The model under review builds one solid part; all positions refer to its coordinate system, in mm. A direction names the side the tool comes from. Coordinates: 2 decimals unless noted, no trailing zeros. Write each loop counter-clockwise with the first axis right and the second up, starting at its lowest first coordinate (ties: lowest second). Pieces come first, ordered by that corner, then holes.
1) For line 1 (Y direction, x = -37, z = 0.65); line 2 (X direction, y = 5.5, z = -1.3); line 3 (X direction, y = 25.5, z = -0.15), list the stretches that pass through material, from the lowest coordinate up.
2) Add section A-A, the plane y = 30. State the section outline as (x, z) points, then the cut area to 3 significant figures.
3) Add section B-B, the plane y = 2.5. State the section outline as (x, z) points.
4) Add section C-C, the plane x = 7. State the section outline as (y, z) points.
5) For P1, Ø1.6, axis at x = 36.5, z = 1, coming from the -Y side; P2, Ø1.5, axis at x = 9, z = -1.5, coming from the -Y side, all flat-tipped, find the tip position at first contact; note any pin that passes through.
6) Machinability: for faces 4 (the cylindrical face through (-46.07, 46, -0.03)), 5 (the flat face through (37, 12.5, 0)), 6 (the flat face through (-35.5, 20, 0)), which of the approach directions +Z, -Z, +X, -X, +Y, -Y give a long, thin tool a straight path to every point of the face, cutting with its end or side? Answer none if there is none.
7) Mouldability with a two-part tool opening along Y and no side actions: class faces 1 (the flat face through (-38, -17.5, 0)), 2 (the flat face through (42, -51.5, 0)), 3 (the flat face through (10.5, 29, 0)) as released by +Y, released by -Y, zero draft, split by the parting line, or undercut.
from build123d import *

# Parameters (mm, degrees)
BOSS_EXTRUDE1_DEPTH = 2
SKETCH2_W           = 10
SKETCH2_H           = 4
BOSS_EXTRUDE2_DEPTH = 4
FILLET1_R           = 5


with BuildPart() as part:
    # Sketch1 → Boss-Extrude1 (new, symmetric)
    with BuildSketch(Plane.XY):
        Polygon((-47.5, -47.5), (-35.5, -47.5), (-35.5, -32.5), (-39.5, -32.5), (-39.5, -17.5), (-35.5, -17.5), (-35.5, -2.5), (-39.5, -2.5), (-39.5, 12.5), (-35.5, 12.5), (-35.5, 27.5), (-25.5, 27.5), (-25.5, 31.5), (-10.5, 31.5), (-10.5, 27.5), (10.5, 27.5), (10.5, 31.5), (25.5, 31.5), (25.5, 27.5), (35.5, 27.5), (35.5, 12.5), (39.5, 12.5), (39.5, -2.5), (35.5, -2.5), (35.5, -17.5), (39.5, -17.5), (39.5, -32.5), (35.5, -32.5), (35.5, -47.5), (47.5, -47.5), (47.5, 47.5), (-47.5, 47.5), align=None)
    extrude(amount=BOSS_EXTRUDE1_DEPTH, both=True)

    # Sketch2 → Boss-Extrude2 (add)
    with BuildSketch(Plane.XZ.offset(47.5)):
        with Locations((-42.5, 0)):
            Rectangle(SKETCH2_W, SKETCH2_H)
        with Locations((42.5, 0)):
            Rectangle(SKETCH2_W, SKETCH2_H)
    extrude(amount=BOSS_EXTRUDE2_DEPTH)

    # Fillet1
    fillet1_edges = [part.edges().sort_by_distance(p)[0] for p in [
        (-47.5, 47.5, 0),
        (47.5, 47.5, 0),
    ]]
    fillet(fillet1_edges, radius=FILLET1_R)


solid = part.part
Geometry results:
1. line 1: y = -47.5 to -32.5, -17.5 to -2.5, 12.5 to 47.5
1. line 2: x = -47.5 to -39.5, 39.5 to 47.5
1. line 3: x = -47.5 to -35.5, 35.5 to 47.5
2. outline: (-47.5, -2) - (-25.5, -2) - (-25.5, 2) - (-47.5, 2) - close; (-10.5, -2) - (10.5, -2) - (10.5, 2) - (-10.5, 2) - close; (25.5, -2) - (47.5, -2) - (47.5, 2) - (25.5, 2) - close
2. area: 260 mm2
3. outline: (-47.5, -2) - (-39.5, -2) - (-39.5, 2) - (-47.5, 2) - close; (39.5, -2) - (47.5, -2) - (47.5, 2) - (39.5, 2) - close
4. outline: (27.5, -2) - (47.5, -2) - (47.5, 2) - (27.5, 2) - close
5. P1: stops at y = -47.5
5. P2: stops at y = 27.5
6. face 4: +Z, -Z, -X, +Y
6. face 5: +Z, -Z
6. face 6: +Z, -Z, -Y
7. face 1: undercut
7. face 2: released by -Y
7. face 3: zero draft
